Here's how the part is built. I have some questions about the finished solid (model axes, mm). Face numbers are marked on the shaded views. A direction names the side the tool comes from. Round coordinates to 2 decimals unless told otherwise and drop trailing zeros. Order: outer loops, then holes, each group sorted by start corner. A loop starts at its lowest first (then second) coordinate and runs counter-clockwise, first axis right, second up. Notation, with made-up numbers: (54, -14) - (97, -14) arc R9 cw to (97, -8) - close; hole circle Ø7 at (23, 5.5). An arc over 180 degrees is marked (long way). Answer as a JSON object with one key per item and string values.
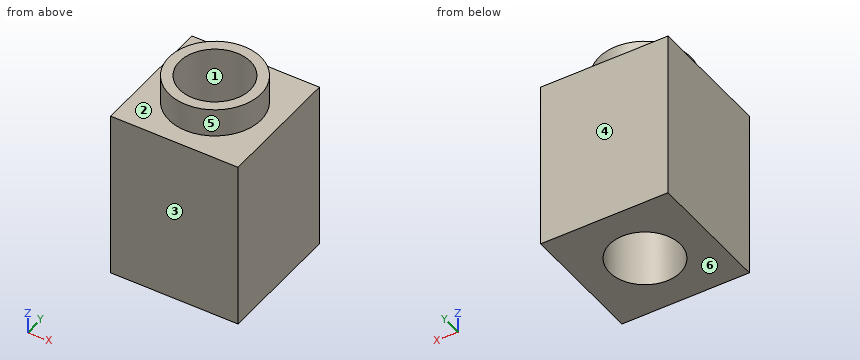
```python
from build123d import *

# Parameters (mm, degrees)
SKETCH_W     = 9
SKETCH_H     = 9
SKETCH_R     = 2.5
PAD_DEPTH    = 12
SKETCH001_R  = 3.25
PAD001_DEPTH = 2
SKETCH002_R  = 2.5
POCKET_DEPTH = 2


with BuildPart() as part:
    # Sketch → Pad (new body)
    with BuildSketch(Plane.XY):
        with Locations((4.5, -4.5)):
            Rectangle(SKETCH_W, SKETCH_H)
        with Locations((4.5, -4.5)):
            Circle(SKETCH_R, mode=Mode.SUBTRACT)
    extrude(amount=PAD_DEPTH)

    # Sketch001 (on Face7 of Pad) → Pad001 (join)
    with BuildSketch(Plane.XY.offset(12)):
        with Locations((4.5, -4.5)):
            Circle(SKETCH001_R)
    extrude(amount=PAD001_DEPTH)

    # Sketch002 (on Face10 of Pad001) → Pocket (cut)
    with BuildSketch(Plane.XY.offset(14)):
        with Locations((4.5, -4.5)):
            Circle(SKETCH002_R)
    extrude(amount=-POCKET_DEPTH, mode=Mode.SUBTRACT)


solid = part.part
```
1. Imagine slicing it at A-A (y = -4.5). List the corners of the cut face in (x, z) for me, plus the area to 3 significant figures.
Responses:
{"outline": "(0, 0) - (2, 0) - (2, 14) - (1.25, 14) - (1.25, 12) - (0, 12) - close; (7, 0) - (9, 0) - (9, 12) - (7.75, 12) - (7.75, 14) - (7, 14) - close", "area": "51.0 mm2"}
2. Imagine slicing it at C-C (x = 7.5). List the corners of the cut face in (y, z) for me.
Responses:
{"outline": "(-9, 0) - (0, 0) - (0, 12) - (-3.25, 12) - (-3.25, 14) - (-5.75, 14) - (-5.75, 12) - (-9, 12) - close"}
3. For the marked faces 5 and 6, which set-ups out of +Z, -Z, +X, -X, +Y, -Y let a thin tool reach every point of the face, with its end or its side?
Responses:
{"face 5": "+Z", "face 6": "-Z, +X, -X, +Y, -Y"}
4. Imagine slicing it at D-D (z = 11). List the corners of the cut face in (x, y) for me, plus the area to 3 significant figures.
Responses:
{"outline": "(0, -9) - (9, -9) - (9, 0) - (0, 0) - close; hole circle Ø5 at (4.5, -4.5)", "area": "61.4 mm2"}
5. If I drill on L1, parallel to Y at x = 4.5, z = 10.5; L2, parallel to X at y = -6.25, z = 3.5; L3, parallel to Y at x = 5.5, z = 3, over which ranges is the centre line in solid material (lowest first)? Write a range as [from, to].
Responses:
{"L1": "[-9, -7], [-2, 0]", "L2": "[0, 2.71], [6.29, 9]", "L3": "[-9, -6.79], [-2.21, 0]"}
6. Thinking about a two-plate mould opening in Y: for the marked faces 1, 2, 3 and 4, which applies, pulls with the +Y half, pulls with the -Y half, needs draft (parallel to the pull), parting line crosses it, or undercut?
Responses:
{"face 1": "undercut", "face 2": "needs draft", "face 3": "pulls with the -Y half", "face 4": "pulls with the +Y half"}
7. Imagine slicing it at B-B (x = 6.25). List the corners of the cut face in (y, z) for me, plus the area to 3 significant figures.
Responses:
{"outline": "(-9, 0) - (-6.29, 0) - (-6.29, 14) - (-7.24, 14) - (-7.24, 12) - (-9, 12) - close; (-2.71, 0) - (0, 0) - (0, 12) - (-1.76, 12) - (-1.76, 14) - (-2.71, 14) - close", "area": "69.0 mm2"}
